Model file for the job. Use its own axes, mm. Face numbers are marked on the shaded views. Coordinates: 2 decimals unless noted, no trailing zeros. Loops run counter-clockwise (first coordinate to the right, second up) from the corner with the lowest first, then second, coordinate; pieces in that order, holes last.
from build123d import *

# Parameters (mm, degrees)
RADYUS1_R = 0.6


with BuildPart() as part:
    # Çizim1 → Döndür1 (revolve)
    with BuildSketch(Plane.XY, mode=Mode.PRIVATE) as d_nd_r1_sk:
        with BuildLine():
            Line((-3.5, 11), (3.5, 11))
            Line((3.5, 11), (3.5, 9.55))
            Line((3.5, 9.55), (2, 9.55))
            ThreePointArc((2, 9.55), (0, 10.313932023), (-2, 9.55))
            Line((-2, 9.55), (-3.5, 9.55))
            Line((-3.5, 9.55), (-3.5, 11))
        make_face()
    revolve(d_nd_r1_sk.sketch.rotate(Axis((-13.551089688, 0, 0), (1, 0, 0)), 90), axis=Axis((-13.551089688, 0, 0), (1, 0, 0)))

    # Radyus1
    radyus1_edges = [part.edges().sort_by_distance(p)[0] for p in [
        (3.5, 0, -11),
        (-3.5, 0, -11),
    ]]
    fillet(radyus1_edges, radius=RADYUS1_R)


solid = part.part
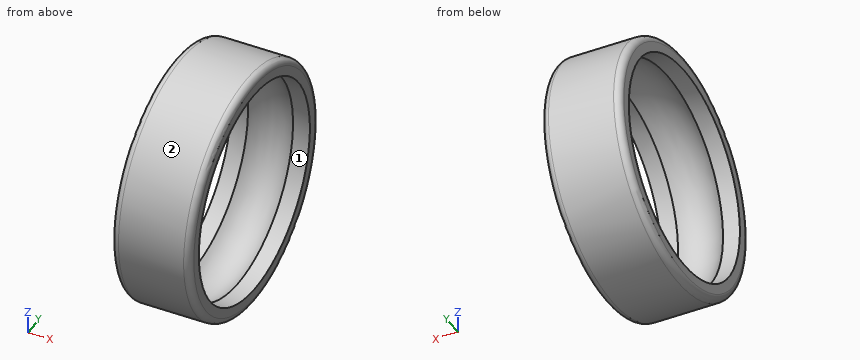
Q1. Drill centre lines: line 1 (Y direction, x = -2.7, z = 0); line 2 (Y direction, x = 3, z = -6.5); line 3 (Z direction, x = 3.25, y = -7.75). Where is each one in solid material? Low to high.
Answers:
line 1: y = -11 to -9.55, 9.55 to 11
line 2: y = -8.86 to -7, 7 to 8.86
line 3: z = -7.65 to -5.58, 5.58 to 7.65
Q2. Slice it at B-B (x = -0.75). List the corners of the cut face in (y, z), and give its area (3 significant figures).
Answers:
outline: circle Ø22 at (0, 0); hole circle Ø20.44 at (0, 0)
area: 52.1 mm2
Q3. Flat gauge pins, fed straight in: P1, Ø2, axis at x = 1, z = -8, coming from the -Y side; P2, Ø1.5, axis at x = 3, y = 6.5, coming from the -Z side; P3, Ø11.5, axis at y = 0, z = 0, coming from the -X side; P4, Ø2, axis at x = 0, z = -3.5, coming from the -Y side. Where does each tip first touch, or does it go through?
Answers:
P1: stops at y = -8.49
P2: stops at z = -9.37
P3: passes through
P4: stops at y = -10.71
Q4. Mould opens along Z. For the marked faces 1 and 2 say: +Z half, -Z half, draft (parallel to the pull), parting line (faces both ways), or undercut.
Answers:
face 1: undercut
face 2: parting line
Q5. Slice it at A-A (z = 0). List the corners of the cut face in (x, y).
Answers:
outline: (-3.5, -10.4) arc R0.6 ccw to (-2.9, -11) - (2.9, -11) arc R0.6 ccw to (3.5, -10.4) - (3.5, -9.55) - (2, -9.55) arc R3 cw to (-2, -9.55) - (-3.5, -9.55) - close; (-3.5, 9.55) - (-2, 9.55) arc R3 cw to (2, 9.55) - (3.5, 9.55) - (3.5, 10.4) arc R0.6 ccw to (2.9, 11) - (-2.9, 11) arc R0.6 ccw to (-3.5, 10.4) - close
